Input: part model. Units: mm. Frame: model coordinates. A direction names the side the tool comes from. Give positions to 0.01 mm unless a question says otherwise; leave off trailing zeros. Loops run counter-clockwise (first coordinate to the right, second up) from the corner with the lowest first, then second, coordinate; pieces in that order, holes last. Notation, with made-up numbers: (25.5, 21) - (54.5, 21) arc R34 ccw to (54.5, 52) - close; hole circle Ø10 at (15.5, 6.5). An arc over 180 degrees is marked (long way). Answer as a JSON object with one key per item and string values.
from build123d import *

# Parameters (mm, degrees)
F0_W     = 266.7
F0_H     = 114.3
F1_DEPTH = 4.7752
F2_W     = 4.7625
F2_H     = 6.35
F2_W_2   = 6.35
F2_H_2   = 4.7625
F3_DEPTH = 38.1
F4_W     = 190.5
F4_H     = 38.1
F4_W_2   = 180.975
F4_H_2   = 28.575
F5_DEPTH = 50.8
F6_W     = 254
F6_H     = 101.6
F6_W_2   = 244.475
F6_H_2   = 92.075
F7_DEPTH = 12.7
F9_DEPTH = 266.7


# Not quite as in the source:
# - a feature names something its author has since deleted; it is built from what else it names


with BuildPart() as f1:
    # F0 (on Top) → F1 (new body)
    with BuildSketch(Plane.XY):
        with Locations((-133.35, -57.15)):
            Rectangle(F0_W, F0_H)
    extrude(amount=F1_DEPTH)

    # F2 (on face) → F3 (join)
    with BuildSketch(Plane.XY.offset(4.7752)):
        with Locations((-257.96875, -104.775)):
            Rectangle(F2_W, F2_H)
        with Locations((-257.96875, -85.725)):
            Rectangle(F2_W, F2_H)
        with Locations((-257.96875, -66.675)):
            Rectangle(F2_W, F2_H)
        with Locations((-257.96875, -47.625)):
            Rectangle(F2_W, F2_H)
        with Locations((-257.96875, -28.575)):
            Rectangle(F2_W, F2_H)
        with Locations((-257.96875, -9.525)):
            Rectangle(F2_W, F2_H)
        with Locations((-238.125, -105.56875)):
            Rectangle(F2_W_2, F2_H_2)
        with Locations((-219.075, -105.56875)):
            Rectangle(F2_W_2, F2_H_2)
        with Locations((-200.025, -105.56875)):
            Rectangle(F2_W_2, F2_H_2)
        with Locations((-180.975, -105.56875)):
            Rectangle(F2_W_2, F2_H_2)
        with Locations((-161.925, -105.56875)):
            Rectangle(F2_W_2, F2_H_2)
        with Locations((-142.875, -105.56875)):
            Rectangle(F2_W_2, F2_H_2)
        with Locations((-123.825, -105.56875)):
            Rectangle(F2_W_2, F2_H_2)
        with Locations((-104.775, -105.56875)):
            Rectangle(F2_W_2, F2_H_2)
        with Locations((-85.725, -105.56875)):
            Rectangle(F2_W_2, F2_H_2)
        with Locations((-66.675, -105.56875)):
            Rectangle(F2_W_2, F2_H_2)
        with Locations((-47.625, -105.56875)):
            Rectangle(F2_W_2, F2_H_2)
        with Locations((-28.575, -105.56875)):
            Rectangle(F2_W_2, F2_H_2)
        with Locations((-8.73125, -104.775)):
            Rectangle(F2_W, F2_H)
        with Locations((-8.73125, -85.725)):
            Rectangle(F2_W, F2_H)
        with Locations((-8.73125, -9.525)):
            Rectangle(F2_W, F2_H)
        with Locations((-8.73125, -28.575)):
            Rectangle(F2_W, F2_H)
        with Locations((-8.73125, -47.625)):
            Rectangle(F2_W, F2_H)
        with Locations((-8.73125, -66.675)):
            Rectangle(F2_W, F2_H)
        with Locations((-123.825, -8.73125)):
            Rectangle(F2_W_2, F2_H_2)
        with Locations((-200.025, -8.73125)):
            Rectangle(F2_W_2, F2_H_2)
        with Locations((-180.975, -8.73125)):
            Rectangle(F2_W_2, F2_H_2)
        with Locations((-28.575, -8.73125)):
            Rectangle(F2_W_2, F2_H_2)
        with Locations((-161.925, -8.73125)):
            Rectangle(F2_W_2, F2_H_2)
        with Locations((-238.125, -8.73125)):
            Rectangle(F2_W_2, F2_H_2)
        with Locations((-85.725, -8.73125)):
            Rectangle(F2_W_2, F2_H_2)
        with Locations((-142.875, -8.73125)):
            Rectangle(F2_W_2, F2_H_2)
        with Locations((-66.675, -8.73125)):
            Rectangle(F2_W_2, F2_H_2)
        with Locations((-219.075, -8.73125)):
            Rectangle(F2_W_2, F2_H_2)
        with Locations((-104.775, -8.73125)):
            Rectangle(F2_W_2, F2_H_2)
        with Locations((-47.625, -8.73125)):
            Rectangle(F2_W_2, F2_H_2)
    extrude(amount=F3_DEPTH)

    # F4 (on face) → F5 (join)
    with BuildSketch(Plane.XY.offset(4.7752)):
        with Locations((-133.35, -57.15)):
            Rectangle(F4_W, F4_H)
        with Locations((-133.35, -57.15)):
            Rectangle(F4_W_2, F4_H_2, mode=Mode.SUBTRACT)
    extrude(amount=F5_DEPTH)

    # F6 (on face) → F7 (join)
    with BuildSketch(Plane.XY.offset(42.8752)):
        with Locations((-133.35, -57.15)):
            Rectangle(F6_W, F6_H)
        with Locations((-133.35, -57.15)):
            Rectangle(F6_W_2, F6_H_2, mode=Mode.SUBTRACT)
    extrude(amount=F7_DEPTH)

    # F8 (on face) → F9 (join, through all)
    with BuildSketch(Plane(origin=(-266.7, 0, 0), x_dir=(0, -1, 0), z_dir=(-1, 0, 0))):
        Polygon((0, 58.7502), (114.3, 58.7502), (57.15, 74.6125), align=None)
        Polygon((6.35, 55.5752), (107.95, 55.5752), (114.3, 55.5752), (114.3, 58.7502), (0, 58.7502), (0, 55.5752), align=None)
    extrude(amount=-F9_DEPTH)


solid = f1.part
Item 1: Cut plane B-B (x = -115.5). Return loops of the section in (y, z).
Geometry check:
{"outline": "(-114.3, 0) - (0, 0) - (0, 4.78) - (-38.1, 4.78) - (-38.1, 55.58) - (-11.11, 55.58) - (-11.11, 42.88) - (-6.35, 42.88) - (-6.35, 55.58) - (0, 55.58) - (0, 58.75) - (-57.15, 74.61) - (-114.3, 58.75) - (-114.3, 55.58) - (-107.95, 55.58) - (-107.95, 42.88) - (-103.19, 42.88) - (-103.19, 55.58) - (-76.2, 55.58) - (-76.2, 4.78) - (-114.3, 4.78) - close; hole (-71.44, 4.78) - (-42.86, 4.78) - (-42.86, 55.58) - (-71.44, 55.58) - close"}
Item 2: Cut plane C-C (y = -16). Return loops of the section in (x, z), then the cut area to 3 significant figures.
Geometry check:
{"outline": "(-266.7, 0) - (0, 0) - (0, 4.78) - (-266.7, 4.78) - close; (-266.7, 55.58) - (-260.35, 55.58) - (-260.35, 42.88) - (-255.59, 42.88) - (-255.59, 55.58) - (-11.11, 55.58) - (-11.11, 42.88) - (-6.35, 42.88) - (-6.35, 55.58) - (0, 55.58) - (0, 63.19) - (-266.7, 63.19) - close", "area": "3,430 mm2"}
Item 3: Material intervals for line 1 (Y direction, x = -225, z = 50.5); line 2 (Y direction, x = -142.5, z = 30); line 3 (Y direction, x = -56, z = 11), sorted ascending. Write a range as [from, to].
Geometry check:
{"line 1": "y = [-107.95, -103.19], [-76.2, -38.1], [-11.11, -6.35]", "line 2": "y = [-107.95, -103.19], [-76.2, -71.44], [-42.86, -38.1], [-11.11, -6.35]", "line 3": "y = [-76.2, -71.44], [-42.86, -38.1]"}
Item 4: Mould query, pull axis X, two halves, no side actions, for faces 1 (the face through (-165.1, -106, 24)), 2 (the face through (-258, -101.6, 24)). Classes: released by +X, released by -X, zero draft, split by the parting line, or undercut.
Geometry check:
{"face 1": "undercut", "face 2": "zero draft"}
Item 5: Cut plane A-A (x = -249.5). Return loops of the section in (y, z), then the cut area to 3 significant figures.
Geometry check:
{"outline": "(-114.3, 0) - (0, 0) - (0, 4.78) - (-114.3, 4.78) - close; (-114.3, 55.58) - (-107.95, 55.58) - (-107.95, 42.88) - (-103.19, 42.88) - (-103.19, 55.58) - (-11.11, 55.58) - (-11.11, 42.88) - (-6.35, 42.88) - (-6.35, 55.58) - (0, 55.58) - (0, 58.75) - (-57.15, 74.61) - (-114.3, 58.75) - close", "area": "1,940 mm2"}
Item 6: Contact query for flat-ended pins moving along their axis: P1, Ø4, axis at x = -132, y = -98.5, coming from the +Z side; P2, Ø8, axis at x = -112.5, z = 29, coming from the -Y side; P3, Ø3, axis at x = -201, z = 12.5, coming from the +Y side; P4, Ø2, axis at x = -231, z = 37.5, coming from the +Y side. Output: stop coordinate, or through.
Geometry check:
{"P1": "stops at z = 63.69", "P2": "stops at y = -76.2", "P3": "stops at y = -6.35", "P4": "passes through"}
Item 7: Cut plane D-D (z = 10). Give the number of separate pieces and of enclosed holes in the cut face, then the cut area to 3 significant figures.
Geometry check:
{"separate pieces": "37", "enclosed holes": "1", "area": "3,180 mm2"}
Item 8: Access query for faces 3 (the face through (-9, -69.85, 24)), 4 (the face through (-158.75, -9, 24)), 5 (the face through (-241.3, -106, 24)). Directions: +Z, -Z, +X, -X, +Y, -Y. A direction counts if a zero-diameter tool reaches every point of the face in a straight line with its end or side. Return the directions, or none.
Geometry check:
{"face 3": "+X", "face 4": "+Y", "face 5": "+Y, -Y"}
